```python
from build123d import *

# Parameters (mm, degrees)
F0_R      = 16
F1_DEPTH  = 50
F2_R      = 3
F3_R      = 16
F4_DEPTH  = 20
F7_DEPTH  = 15
F8_W      = 60
F8_H      = 10
F9_DEPTH  = 70
F10_R     = 29.99999
F11_R     = 10
F11_R_2   = 6
F12_DEPTH = 10
F13_DEPTH = 10.001


# Not quite as in the source:
# - a fillet or chamfer is up to 0.001 mm smaller than in the source, because OpenCascade refuses the exact size


with BuildPart() as f1:
    # F0 (on Top) → F1 (new body)
    with BuildSketch(Plane.XY):
        with Locations((-41.7741946876, 23.8037649542)):
            Circle(F0_R)
    extrude(amount=F1_DEPTH)

    # F2
    f2_edges = [f1.edges().sort_by_distance(p)[0] for p in [
        (-57.774195, 23.803765, 0),
    ]]
    fillet(f2_edges, radius=F2_R)

    # F3 (on face) → F4 (join)
    with BuildSketch(Plane.XY.offset(50)):
        with BuildLine():
            Line((-11.7741946876, 58.8037649542), (-41.7741946876, 58.8037649542))
            Line((-41.7741946876, 58.8037649542), (-71.7741946876, 58.8037649542))
            Line((-71.7741946876, 58.8037649542), (-71.7741946876, 23.8037649542))
            Line((-71.7741946876, 23.8037649542), (-71.7741946876, -6.1962350458))
            ThreePointArc((-71.7741946876, -6.1962350458), (-70.3097285935, -9.7317689517), (-66.7741946876, -11.1962350458))
            Line((-66.7741946876, -11.1962350458), (-56.7741946876, -11.1962350458))
            Line((-56.7741946876, -11.1962350458), (-41.7741946876, -11.1962350458))
            Line((-41.7741946876, -11.1962350458), (-26.7741946876, -11.1962350458))
            Line((-26.7741946876, -11.1962350458), (-16.7741946876, -11.1962350458))
            ThreePointArc((-16.7741946876, -11.1962350458), (-13.2386607817, -9.7317689517), (-11.7741946876, -6.1962350458))
            Line((-11.7741946876, -6.1962350458), (-11.7741946876, 58.8037649542))
        make_face()
        with Locations((-41.7741946876, 23.8037649542)):
            Circle(F3_R, mode=Mode.SUBTRACT)
        with Locations((-41.7741946876, 23.8037649542)):
            Circle(F3_R)
    extrude(amount=F4_DEPTH)

    # F6 (on offset) → F7 (cut, symmetric)
    with BuildSketch(Plane(origin=(-41.7741946876, 0, 0), x_dir=(0, -1, 0), z_dir=(-1, 0, 0))):
        Polygon((11.2580982968, 59.3282932557), (11.2580982968, 70.0462609529), (-28.7419017032, 70.0462609529), align=None)
    extrude(amount=F7_DEPTH, both=True, mode=Mode.SUBTRACT)

    # F8 (on face) → F9 (join)
    with BuildSketch(Plane.XY.offset(70)):
        with Locations((-41.7741946876, 53.8037649542)):
            Rectangle(F8_W, F8_H)
    extrude(amount=F9_DEPTH)

    # F10 (radius 30 in the source; OpenCascade refuses exactly that, so slightly less here)
    f10_edges = [f1.edges().sort_by_distance(p)[0] for p in [
        (-71.774195, 53.803765, 140),
        (-11.774195, 53.803765, 140),
    ]]
    fillet(f10_edges, radius=F10_R)

    # F11 (on face) → F12 (join)
    with BuildSketch(Plane.XZ.offset(-48.8037649542)):
        with Locations((-41.7741946876, 110)):
            Circle(F11_R)
        with Locations((-41.7741946876, 110)):
            Circle(F11_R_2, mode=Mode.SUBTRACT)
    extrude(amount=F12_DEPTH)

    # F13 (cut, through all): a face of the model
    f13_faces = [f1.faces().sort_by_distance(p)[0] for p in [
        (-41.7741946876, 48.8037649542, 110),
    ]]
    extrude(f13_faces, amount=-F13_DEPTH, mode=Mode.SUBTRACT)


solid = f1.part
```
Here's how the part is built. I have some questions about the finished solid (model axes, mm). A direction names the side the tool comes from. Coordinates: 2 decimals unless noted, no trailing zeros. Order: outer loops, then holes, each group sorted by start corner. A loop starts at its lowest first (then second) coordinate and runs counter-clockwise, first axis right, second up.
1) Imagine slicing it at B-B on z = 106. List the corners of the cut face in (x, y) for me.
2) Will these pins go through, and if not, where does the flat tip stop? pin 1 (2 mm diameter, centred on x = -47, y = 31, fed in from +Z); pin 2 (9.5 mm diameter, centred on x = -41.77, z = 110, fed in from +Y); pin 3 (12 mm diameter, centred on y = 8, z = 27, fed in from +X); pin 4 (15.5 mm diameter, centred on x = -41.77, z = 110, fed in from -Y).
3) Which directions (+Z, -Z, +X, -X, +Y, -Y) give clear straight access to the entire face, cutting with the end or side of a thin tool? Please do faces 5 (the face through (-26.774, 0, 67)), 6 (the face through (-56, 32, 50)), 7 (the face through (-43.076, 43.874, 119.915)), 8 (the face through (-13.28, -9.77, 59.86)).
4) We'd pull the mould along X, two halves only. Please class faces 1 (the face through (-41.984, 8.965, 64.747)), 2 (the face through (-63.2, 53.9, 131)), 3 (the face through (-56.774, 0, 67)), 4 (the face through (-37, 38.804, 106)): +X half, -X half, draft (parallel to the pull), parting line (faces both ways), or undercut.
5) I need wall thicknesses on line 1 (Z direction, x = -15.5, y = 38.5); line 2 (Y direction, x = -58.5, z = 122); line 3 (Z direction, x = -45, y = 47). Which ranges of each line are inside material? Lowest first, please.
6) Imagine slicing it at D-D on z = 77. List the corners of the cut face in (x, y) for me, and give its area (3 significant figures).
7) Imagine slicing it at C-C on x = -62.5. List the corners of the cut face in (y, z) for me.
Response values:
1. outline: (-71.77, 48.8) - (-50.94, 48.8) - (-50.94, 38.8) - (-46.25, 38.8) - (-46.25, 58.8) - (-71.77, 58.8) - close; (-37.3, 38.8) - (-32.61, 38.8) - (-32.61, 48.8) - (-11.77, 48.8) - (-11.77, 58.8) - (-37.3, 58.8) - close
2. pin 1: stops at z = 70
2. pin 2: passes through
2. pin 3: stops at x = -29.13
2. pin 4: stops at y = 38.8
3. face 5: +Z, -Y
3. face 6: -Z
3. face 7: -Y
3. face 8: +Z, -Z, +X, -Y
4. face 1: undercut
4. face 2: -X half
4. face 3: undercut
4. face 4: draft
5. line 1: z = 50 to 70
5. line 2: y = 48.8 to 58.8
5. line 3: z = 50 to 70, 100.53 to 104.94, 115.06 to 119.47
6. outline: (-71.77, 48.8) - (-11.77, 48.8) - (-11.77, 58.8) - (-71.77, 58.8) - close
6. area: 600 mm2
7. outline: (-11.2, 50) - (58.8, 50) - (58.8, 131.69) - (48.8, 131.69) - (48.8, 70) - (-11.2, 70) - close
